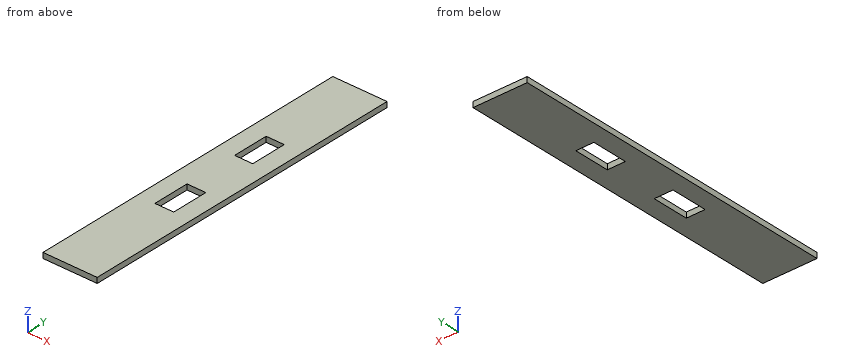
```python
from build123d import *

# Parameters (mm, degrees)
CROQUIS1_W              = 150
CROQUIS1_H              = 920
SALIENTE_EXTRUIR1_DEPTH = 15
CROQUIS3_W              = 52
CROQUIS3_H              = 102
CORTAR_EXTRUIR1_DEPTH   = 200
CROQUIS7_W              = 50
CROQUIS7_H              = 100
CORTAR_EXTRUIR2_DEPTH   = 467.315343947


with BuildPart() as part:
    # Croquis1 → Saliente-Extruir1 (new body)
    with BuildSketch(Plane.XY):
        Rectangle(CROQUIS1_W, CROQUIS1_H)
    extrude(amount=SALIENTE_EXTRUIR1_DEPTH)

    # Croquis3 → Cortar-Extruir1 (cut, symmetric)
    with BuildSketch(Plane(origin=(0, 0, 0), x_dir=(-1, 0, 0), z_dir=(0, 0, -1))):
        with Locations((0, -110)):
            Rectangle(CROQUIS3_W, CROQUIS3_H)
    extrude(amount=CORTAR_EXTRUIR1_DEPTH, both=True, mode=Mode.SUBTRACT)

    # Croquis7 → Cortar-Extruir2 (cut, through all)
    with BuildSketch(Plane(origin=(0, 0, 0), x_dir=(-1, 0, 0), z_dir=(0, 0, -1))):
        with Locations((0, 141)):
            Rectangle(CROQUIS7_W, CROQUIS7_H)
    extrude(amount=-CORTAR_EXTRUIR2_DEPTH, mode=Mode.SUBTRACT)


solid = part.part
```
The model under review builds one solid part; all positions refer to its coordinate system, in mm. Round coordinates to 2 decimals unless told otherwise and drop trailing zeros. Write each loop counter-clockwise with the first axis right and the second up, starting at its lowest first coordinate (ties: lowest second). Pieces come first, ordered by that corner, then holes.
(1) We need section B-B on x = 7. Give the boundary of the cut face in (y, z).
(2) We need section C-C on z = 9. Give the boundary of the cut face in (x, y), and give its area (3 significant figures).
(3) Wall thickness on L1, parallel to Y at x = 22.5, z = 13; L2, parallel to X at y = -157, z = 7: over which ranges is each line inside the solid? List them lowest first.
(4) We need section D-D on y = -68.5. Give the boundary of the cut face in (x, z), and give its area (3 significant figures).
(5) Insertion check: pin 1 (4 mm diameter, centred on x = 41, y = 233.5, fed in from -Z). The pin has a flat end and moves straight along its axis. Give the tip position at first contact, or say it passes through.
(6) We need section A-A on y = 128. Give the boundary of the cut face in (x, z).
Findings below:
1. outline: (-460, 0) - (-161, 0) - (-161, 15) - (-460, 15) - close; (-59, 0) - (91, 0) - (91, 15) - (-59, 15) - close; (191, 0) - (460, 0) - (460, 15) - (191, 15) - close
2. outline: (-75, -460) - (75, -460) - (75, 460) - (-75, 460) - close; hole (-26, -161) - (26, -161) - (26, -59) - (-26, -59) - close; hole (-25, 91) - (25, 91) - (25, 191) - (-25, 191) - close
2. area: 128,000 mm2
3. L1: y = -460 to -161, -59 to 91, 191 to 460
3. L2: x = -75 to -26, 26 to 75
4. outline: (-75, 0) - (-26, 0) - (-26, 15) - (-75, 15) - close; (26, 0) - (75, 0) - (75, 15) - (26, 15) - close
4. area: 1,470 mm2
5. pin 1: stops at z = 0
6. outline: (-75, 0) - (-25, 0) - (-25, 15) - (-75, 15) - close; (25, 0) - (75, 0) - (75, 15) - (25, 15) - close
